Geometry check sheet. Reference: the model listing, model coordinates, mm. Face numbers are marked on the shaded views. A direction names the side the tool comes from. Coordinates: 2 decimals unless noted, no trailing zeros. Order: outer loops, then holes, each group sorted by start corner. A loop starts at its lowest first (then second) coordinate and runs counter-clockwise, first axis right, second up. Notation, with made-up numbers: (-23.75, 12.25) - (-1.75, 12.25) arc R32 cw to (-1.75, 40.25) - close; hole circle Ø2 at (-18.5, -24.75). An arc over 180 degrees is marked (long way). Return JSON: item names as keys, results as strings. Group by question number.
Item 1: Draft check along Y on the marked faces 1, 2, 3 and 4. Enter one of: pulls with the +Y half, pulls with the -Y half, needs draft (parallel to the pull), parting line crosses it, or undercut.
Item 2: Section check A-A on x = 1. Enter the section's corners in (y, z), then the cut area to 3 significant figures.
Item 3: Scan lines: probe 1 along Y at (x, z) = (-0.75, -31.75); probe 2 along Y at (x, z) = (1.75, 3.5); probe 3 along Z at (x, y) = (2.5, -0.5). Record each from-to range of solid material in increasing order.
Item 4: Gauge pin test, flat end, axial feed: pin 1 (1.8 mm diameter, centred on x = 0, y = -2, fed in from +Z). Record the tip position at first contact, or that the pin passes through.
Item 5: Section check C-C on y = 0. Enter the section's corners in (x, z), then the cut area to 3 significant figures.
Item 6: Section check D-D on y = -13.5. Enter the section's corners in (x, z).
Item 7: Tool access check on the marked faces 5, 6 and 7. Record the directions out of +Z, -Z, +X, -X, +Y, -Y that give a thin tool (end or side, any length) a straight path to the whole face; none if there is none.
Item 8: Section check B-B on z = 1.5. Enter the section's corners in (x, y).
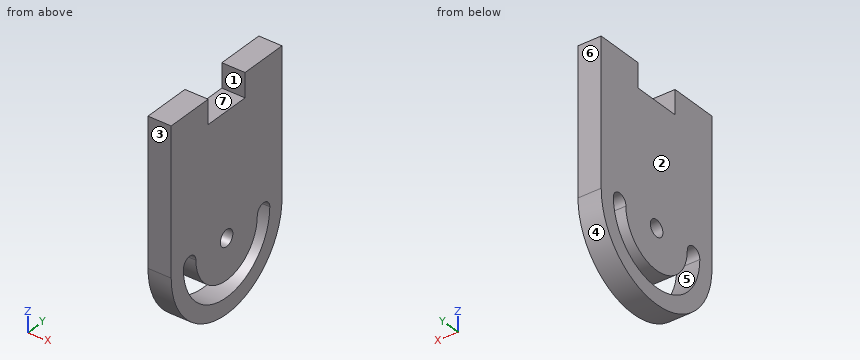
from build123d import *

# Parameters (mm, degrees)
BOSS_EXTRUDE1_DEPTH   = 3.048
F_8_CLEARANCE_HOLE1_D = 4.3053
CUT_EXTRUDE1_DEPTH    = 55.595821415


with BuildPart() as part:
    # Sketch1 → Boss-Extrude1 (new, symmetric)
    with BuildSketch(Plane(origin=(0, 0, 0), x_dir=(0, 0, -1), z_dir=(1, 0, 0))):
        with BuildLine():
            Line((0, 6.35), (0, -6.35))
            Line((0, -6.35), (-6.35, -6.35))
            Line((-6.35, -6.35), (-6.35, -19.05))
            Line((-6.35, -19.05), (31.75, -19.05))
            ThreePointArc((31.75, -19.05), (50.8, 0), (31.75, 19.05))
            Line((31.75, 19.05), (-6.35, 19.05))
            Line((-6.35, 19.05), (-6.35, 6.35))
            Line((-6.35, 6.35), (0, 6.35))
        make_face()
    extrude(amount=BOSS_EXTRUDE1_DEPTH, both=True)

    # #8 Clearance Hole1 (through all)
    with Locations(Plane(origin=(3.048, 0, 0), x_dir=(0, 0, -1), z_dir=(1, 0, 0))):
        with Locations((31.75, 0), (31.75, 12.7), (31.75, -12.7)):
            Hole(F_8_CLEARANCE_HOLE1_D / 2)

    # Sketch5 → Cut-Extrude1 (cut, through all)
    with BuildSketch(Plane(origin=(3.048, 0, 0), x_dir=(0, 0, -1), z_dir=(1, 0, 0))):
        with BuildLine():
            ThreePointArc((33.90265, 12.7), (33.272153413, 11.177846587), (31.75, 10.54735))
            ThreePointArc((31.75, 10.54735), (42.29735, 0), (31.75, -10.54735))
            ThreePointArc((31.75, -10.54735), (33.272153413, -11.177846587), (33.90265, -12.7))
            ThreePointArc((33.90265, -12.7), (33.272153413, -14.222153413), (31.75, -14.85265))
            ThreePointArc((31.75, -14.85265), (46.60265, 0), (31.75, 14.85265))
            ThreePointArc((31.75, 14.85265), (33.272153413, 14.222153413), (33.90265, 12.7))
        make_face()
    extrude(amount=-CUT_EXTRUDE1_DEPTH, mode=Mode.SUBTRACT)


solid = part.part
Computed:
{
 "1": {"face 1": "undercut", "face 2": "needs draft", "face 3": "pulls with the -Y half", "face 4": "parting line crosses it"},
 "2": {"outline": "(-19.05, -31.75) arc R19.05 ccw to (19.05, -31.75) - (19.05, 6.35) - (6.35, 6.35) - (6.35, 0) - (-6.35, 0) - (-6.35, 6.35) - (-19.05, 6.35) - close; hole (-14.85, -31.75) arc R14.85 ccw to (14.85, -31.75) arc R2.15 ccw to (10.55, -31.75) arc R10.55 cw to (-10.55, -31.75) arc R2.15 ccw to start; hole circle Ø4.31 at (0, -31.75)", "area": "1,740 mm²"},
 "3": {"probe 1": "y = -19.05 to -14.85, -10.55 to -2.15, 2.15 to 10.55, 14.85 to 19.05", "probe 2": "y = -19.05 to -6.35, 6.35 to 19.05", "probe 3": "z = -50.79 to -46.59, -42.29 to -33.84, -29.66 to 0"},
 "4": {"pin 1": "stops at z = 0"},
 "5": {"outline": "(-3.05, -50.8) - (3.05, -50.8) - (3.05, -46.6) - (-3.05, -46.6) - close; (-3.05, -42.3) - (3.05, -42.3) - (3.05, -33.9) - (-3.05, -33.9) - close; (-3.05, -29.6) - (3.05, -29.6) - (3.05, 0) - (-3.05, 0) - close", "area": "257 mm²"},
 "6": {"outline": "(-3.05, -45.19) - (3.05, -45.19) - (3.05, -37.94) - (-3.05, -37.94) - close; (-3.05, -29.75) - (3.05, -29.75) - (3.05, 6.35) - (-3.05, 6.35) - close"},
 "7": {"face 5": "+X, -X", "face 6": "+Z, -Z, +X, -X, +Y", "face 7": "+Z, +X, -X"},
 "8": {"outline": "(-3.05, -19.05) - (3.05, -19.05) - (3.05, -6.35) - (-3.05, -6.35) - close; (-3.05, 6.35) - (3.05, 6.35) - (3.05, 19.05) - (-3.05, 19.05) - close"}
}
